Here's how the part is built. I have some questions about the finished solid (model axes, mm). Round coordinates to 2 decimals unless told otherwise and drop trailing zeros. Write each loop counter-clockwise with the first axis right and the second up, starting at its lowest first coordinate (ties: lowest second). Pieces come first, ordered by that corner, then holes. Notation, with made-up numbers: (-31, 27.5) -> (-11, 27.5) arc R20 cw to (-11, 66.5) -> close; hole circle Ø5 at (89, 4). An arc over 180 degrees is marked (long way). Answer in a Markdown table with one row per item. Add a question column.
from build123d import *

# Parameters (mm, degrees)
SALIENTE_EXTRUIR1_DEPTH = 620
CROQUIS2_W              = 203.452350599
CROQUIS2_H              = 590
CORTAR_EXTRUIR1_DEPTH   = 117.511998831
CROQUIS3_W              = 213.451905324
CROQUIS3_H              = 600
CORTAR_EXTRUIR2_DEPTH   = 3


with BuildPart() as part:
    # Croquis1 → Saliente-Extruir1 (new body)
    with BuildSketch(Plane.XY):
        Polygon((0, 0), (160, 150), (160, 160), (-10, 0), align=None)
    extrude(amount=SALIENTE_EXTRUIR1_DEPTH)

    # Croquis2 → Cortar-Extruir1 (cut, through all)
    with BuildSketch(Plane(origin=(-4.697247706, 4.990825688, 0), x_dir=(0.728199993, 0.685364699, 0), z_dir=(-0.685364699, 0.728199993, 0))):
        with Locations((109.444175373, -310)):
            Rectangle(CROQUIS2_W, CROQUIS2_H)
    extrude(amount=-CORTAR_EXTRUIR1_DEPTH, mode=Mode.SUBTRACT)

    # Croquis3 → Cortar-Extruir2 (cut)
    with BuildSketch(Plane(origin=(0, 0, 0), x_dir=(0.729537204, 0.683941129, 0), z_dir=(0.683941129, -0.729537204, 0))):
        with Locations((109.430580621, 310)):
            Rectangle(CROQUIS3_W, CROQUIS3_H)
    extrude(amount=-CORTAR_EXTRUIR2_DEPTH, mode=Mode.SUBTRACT)


solid = part.part
Item 1: I need wall thicknesses on line 1 along Z through (x, y) = (78, 82.5); line 2 along Y through (x, z) = (-3, 129.5); line 3 along X through (y, z) = (6.5, 583.5). Which ranges of each line are inside material? Lowest first, please. Write a range as from..to.
Item 2: If we section it at B-B on x = 64: Please give me the cut outline in (y, z).
Item 3: If we mould it in two halves opening along Z, with no side actions, what happens to faces 1 (the flat face through (75, 74, 0)), 2 (the flat face through (160, 155, 306)), 3 (the flat face through (78, 75, 10))? For each: pulls with the +Z half, pulls with the -Z half, needs draft (parallel to the pull), parting line crosses it, or undercut.
Item 4: If we section it at A-A on z = 414: Please give me the cut outline in (x, y).
Results list:
| question | item | result |
|---|---|---|
| 1 | line 1 | 0..15, 605..620 |
| 1 | line 2 | 0..6.59 |
| 1 | line 3 | -3.09..2.55 |
| 2 | outline | (60, 0) -> (69.65, 0) -> (69.65, 15) -> (64.11, 15) -> (64.11, 10) -> (60, 10) -> close; (60, 610) -> (64.11, 610) -> (64.11, 605) -> (69.65, 605) -> (69.65, 620) -> (60, 620) -> close |
| 3 | face 1 | pulls with the -Z half |
| 3 | face 2 | needs draft |
| 3 | face 3 | undercut |
| 4 | outline | (-10, 0) -> (0, 0) -> (1.97, 1.85) -> (-0.08, 4.04) -> (3.57, 7.46) -> (0.92, 10.28) -> close; (149.08, 149.72) -> (152, 146.61) -> (155.64, 150.03) -> (157.69, 147.84) -> (160, 150) -> (160, 160) -> close |
